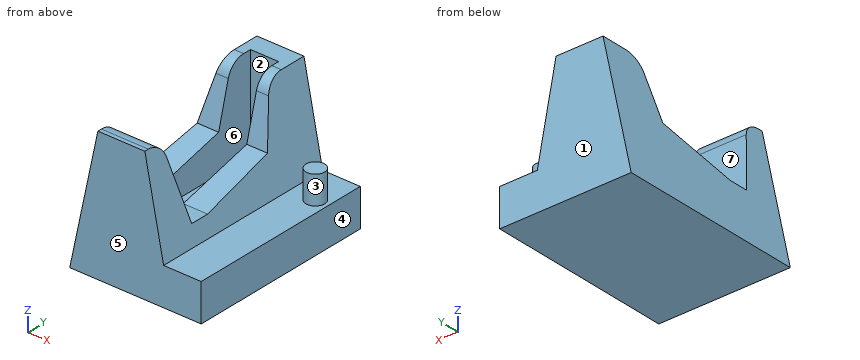
```python
from build123d import *

# Parameters (mm, degrees)
F1_DEPTH = 100
F3_DEPTH = 70.001
F4_R     = 10
F5_W     = 15
F5_H     = 60
F6_DEPTH = 50
F7_R     = 5
F8_DEPTH = 15


with BuildPart() as f1:
    # F0 (on Front) → F1 (new body)
    with BuildSketch(Plane.XZ):
        Polygon((15, 70), (0, 0), (70, 0), (70, 20), (50, 20), (40, 70), align=None)
    extrude(amount=-F1_DEPTH)

    # F2 (on face) → F3 (cut, through all)
    with BuildSketch(Plane.YZ.offset(70)):
        Polygon((78.038476, 70), (10, 70), (20, 30), (30, 30), (70, 40), align=None)
    extrude(amount=-F3_DEPTH, mode=Mode.SUBTRACT)

    # F4
    f4_edges = [f1.edges().sort_by_distance(p)[0] for p in [
        (27.5, 10, 70),
        (27.5, 78.038476, 70),
    ]]
    fillet(f4_edges, radius=F4_R)

    # F5 (on face) → F6 (cut)
    with BuildSketch(Plane.XY.offset(70)):
        with Locations((27.5, 60)):
            Rectangle(F5_W, F5_H)
    extrude(amount=-F6_DEPTH, mode=Mode.SUBTRACT)

    # F7 (on face) → F8 (join)
    with BuildSketch(Plane.XY.offset(20)):
        with Locations((63, 80)):
            Circle(F7_R)
    extrude(amount=F8_DEPTH)


solid = f1.part
```
Design review of the part built by this model. Coordinates are the model's own, in mm. Face numbers are marked on the shaded views. A direction names the side the tool comes from. Coordinates: 2 decimals unless noted, no trailing zeros. Order: outer loops, then holes, each group sorted by start corner. A loop starts at its lowest first (then second) coordinate and runs counter-clockwise, first axis right, second up. Notation, with made-up numbers: M 66,39.5 L 106,39.5 A29 ccw 106,60.5 Z; hole C 78.25,86 d9. An arc over 180 degrees is marked long. Answer as a JSON object with one key per item and string values. Group by question number.
1) Wall thickness on L1, parallel to Z at x = 20.5, y = 84; L2, parallel to X at y = 60, z = 20.5; L3, parallel to Z at x = 11, y = 21: over which ranges is each line inside the solid? List them lowest first.
2) Mouldability with a two-part tool opening along X and no side actions: class the marked faces 1, 2, 3 and 4 as pulls with the +X half, pulls with the -X half, needs draft (parallel to the pull), parting line crosses it, or undercut.
3) For pin 1 (5 mm diameter, centred on x = 62.5, y = 79.5, fed in from +Z); pin 2 (1 mm diameter, centred on x = 20, y = 51.5, fed in from +Z); pin 3 (10 mm diameter, centred on x = 56.5, y = 16.5, fed in from +Z); pin 4 (12 mm diameter, centred on x = 25.5, z = 43.5, fed in from -Y), all flat-tipped, find the tip position at first contact; note any pin that passes through.
4) Add section D-D, the plane x = 33.5. Write out the cut boundary in (y, z), then the cut area to 3 significant figures.
5) Tool access review of the marked faces 5, 6 and 7: name each direction out of +Z, -Z, +X, -X, +Y, -Y from which nothing blocks a thin tool from reaching the whole face with its end or side.
6) Add section B-B, the plane z = 33. Write out the cut boundary in (x, y), then the cut area to 3 significant figures.
7) Add section A-A, the plane x = 66. Write out the cut boundary in (y, z), then the cut area to 3 significant figures.
8) Add section C-C, the plane y = 24. Write out the cut boundary in (x, z).
Computed values:
{
 "1": {"L1": "z = 0 to 20", "L2": "x = 4.39 to 20, 35 to 49.9", "L3": "z = 0 to 30"},
 "2": {"face 1": "needs draft", "face 2": "undercut", "face 3": "undercut", "face 4": "pulls with the +X half"},
 "3": {"pin 1": "stops at z = 35", "pin 2": "stops at z = 35.5", "pin 3": "stops at z = 20", "pin 4": "stops at y = 0"},
 "4": {"outline": "M 0,0 L 100,0 L 100,70 L 90,70 L 90,20 L 30,20 L 30,30 L 20,30 L 11.89,62.43 A10 ccw 2.19,70 L 0,70 Z", "area": "3,390 mm^2"},
 "5": {"face 5": "+Z, -Z, +X, -X, -Y", "face 6": "+Z", "face 7": "+Z, +X, -X"},
 "6": {"outline": "M 7.07,0 L 47.4,0 L 47.4,19.25 L 7.07,19.25 Z; M 7.07,42 L 20,42 L 20,90 L 35,90 L 35,42 L 47.4,42 L 47.4,100 L 7.07,100 Z; C 63,80 d10", "area": "2,470 mm^2"},
 "7": {"outline": "M 0,0 L 100,0 L 100,20 L 84,20 L 84,35 L 76,35 L 76,20 L 0,20 Z", "area": "2,120 mm^2"},
 "8": {"outline": "M 0,0 L 70,0 L 70,20 L 50,20 L 48,30 L 6.43,30 Z"}
}
